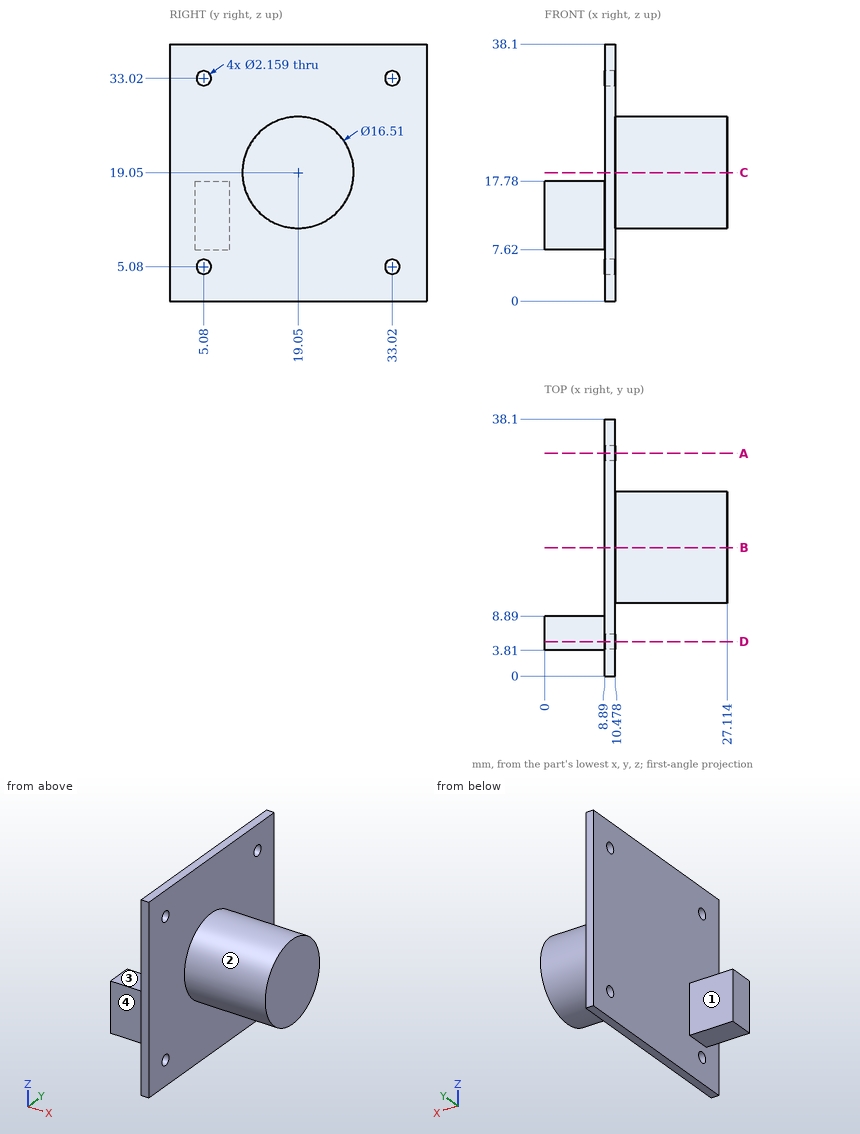
Can you work these out from the drawing? Everything is in mm from the part's minimum corner. A direction names the side the tool comes from. Round coordinates to 2 decimals unless told otherwise and drop trailing zeros. Loops run counter-clockwise (first coordinate to the right, second up) from the corner with the lowest first, then second, coordinate; pieces in that order, holes last. Notation, with made-up numbers: (29, 15.5) -> (61, 15.5) arc R32 cw to (61, 44.5) -> close; hole circle Ø5 at (89, 53). An arc over 180 degrees is marked (long way). Use CSV: the item, a comma, the result in double quotes.
(1) Suppose I cut it at B-B on y = 19.05. Write out the boundary of the cut face in (x, z) (1 decimal), plus the area to 3 significant figures.
Return value:
outline,"(8.9, 0) -> (10.5, 0) -> (10.5, 10.8) -> (27.1, 10.8) -> (27.1, 27.3) -> (10.5, 27.3) -> (10.5, 38.1) -> (8.9, 38.1) -> close"
area,"335 mm²"
(2) Suppose I cut it at D-D on y = 5.08. Write out the boundary of the cut face in (x, z).
Return value:
outline,"(0, 7.62) -> (8.89, 7.62) -> (8.89, 6.16) -> (10.48, 6.16) -> (10.48, 31.94) -> (8.89, 31.94) -> (8.89, 17.78) -> (0, 17.78) -> close; (8.89, 0) -> (10.48, 0) -> (10.48, 4) -> (8.89, 4) -> close; (8.89, 34.1) -> (10.48, 34.1) -> (10.48, 38.1) -> (8.89, 38.1) -> close"
(3) For the marked faces 1, 2, 3 and 4, which set-ups out of +Z, -Z, +X, -X, +Y, -Y let a thin tool reach every point of the face, with its end or its side?
Return value:
face 1,"+Z, -Z, -X, +Y"
face 2,"+X"
face 3,"+Z, -X, +Y, -Y"
face 4,"+Z, -Z, -X, -Y"
(4) Will these pins go through, and if not, where does the flat tip stop? pin 1 Ø4 at (y, z) = (33.5, 14) entering from -X; pin 2 Ø2.5 at (x, z) = (6, 14) entering from -Y; pin 3 Ø3 at (x, y) = (24, 16) entering from +Z.
Return value:
pin 1,"stops at x = 8.89"
pin 2,"stops at y = 3.81"
pin 3,"stops at z = 27.16"
(5) If I drill on probe 1 along Y at (x, z) = (9.85, 5.08); probe 2 along Y at (x, z) = (10, 4.5), over which ranges is the centre line in solid material (lowest first)? Write a range as [from, to].
Return value:
probe 1,"y = [0, 4], [6.16, 31.94], [34.1, 38.1]"
probe 2,"y = [0, 4.17], [5.99, 32.11], [33.93, 38.1]"
(6) Suppose I cut it at A-A on y = 33.02. Write out the boundary of the cut face in (x, z).
Return value:
outline,"(8.89, 0) -> (10.48, 0) -> (10.48, 4) -> (8.89, 4) -> close; (8.89, 6.16) -> (10.48, 6.16) -> (10.48, 31.94) -> (8.89, 31.94) -> close; (8.89, 34.1) -> (10.48, 34.1) -> (10.48, 38.1) -> (8.89, 38.1) -> close"
